The model under review builds one solid part; all positions refer to its coordinate system, in mm. Round coordinates to 2 decimals unless told otherwise and drop trailing zeros. Write each loop counter-clockwise with the first axis right and the second up, starting at its lowest first coordinate (ties: lowest second). Pieces come first, ordered by that corner, then holes. Notation, with made-up numbers: M 57.25,-9 L 92.25,-9 A20 cw 92.25,26 Z; hole C 70.25,-31 d6. An arc over 180 degrees is marked long. Write item = value, one per line. Start each with the question number.
Item 1: Take a section at B-B, the plane z = 4. Give the boundary of the cut face in (x, y), plus the area to 3 significant figures.
Item 2: Take a section at D-D, the plane y = 58.5. Give the boundary of the cut face in (x, z).
Item 3: To check wall thickness, follow line 1 along Z through (x, y) = (70.5, 58.5); line 2 along Z through (x, y) = (70.5, 59); line 3 along Y through (x, z) = (72, 4.5). State the ranges of each line that lie inside material, in increasing order.
Item 4: Take a section at C-C, the plane x = 71.25. Give the number of separate pieces and of enclosed holes in the cut face, plus the area to 3 significant figures.
Item 5: Take a section at A-A, the plane y = 52. Give the boundary of the cut face in (x, z).
Item 6: The part is to be moulded in two halves that separate along Z. For faces 1 (the cylindrical face through (70.04, 78.54, 4.95)), 2 (the flat face through (70, 65, 0)), 3 (the cylindrical face through (70.04, 67.16, 5.06)), say which applies: +Z half, -Z half, draft (parallel to the pull), parting line (faces both ways), or undercut.
Item 7: For pin 1 Ø1.5 at (x, z) = (71.5, 2) entering from +Y; pin 2 Ø1.4 at (x, y) = (71.08, 72.9) entering from +Z; pin 3 Ø3 at (x, z) = (70.5, 2) entering from +Y; pin 4 Ø1.5 at (y, z) = (75, 3) entering from +X, all flat-tipped, find the tip position at first contact; note any pin that passes through.
from build123d import *

# Parameters (mm, degrees)
SKETCH1_R           = 1.2065
BOSS_EXTRUDE1_DEPTH = 10.033
CUT_EXTRUDE1_DEPTH  = 10.033
CUT_EXTRUDE2_DEPTH  = 10.033


with BuildPart() as part:
    # Sketch1 → Boss-Extrude1 (new body)
    with BuildSketch(Plane.XY):
        with BuildLine():
            Line((74.127846298, 88.795942837), (72.00043944, 36.574422097))
            ThreePointArc((72.00043944, 36.574422097), (66.89810991, 60.973237803), (68.966334727, 85.813898433))
            ThreePointArc((68.966334727, 85.813898433), (71.21567331, 87.878558548), (74.127846298, 88.795942837))
        make_face()
        with Locations((70.925382829, 77.722422097)):
            Circle(SKETCH1_R, mode=Mode.SUBTRACT)
        with Locations((71.077782829, 72.896422097)):
            Circle(SKETCH1_R, mode=Mode.SUBTRACT)
    extrude(amount=BOSS_EXTRUDE1_DEPTH)

    # Sketch2 → Cut-Extrude1 (cut)
    with BuildSketch(Plane(origin=(70.393641123, -2.867704976, 0), x_dir=(0, 0, -1), z_dir=(0.999171234, -0.040704363, 0))):
        with BuildLine():
            Line((-1.27, 39.474842481), (-8.763, 39.474842481))
            Line((-8.763, 39.474842481), (-6.9215, 68.049842481))
            ThreePointArc((-6.9215, 68.049842481), (-5.0165, 69.954842481), (-3.1115, 68.049842481))
            Line((-3.1115, 68.049842481), (-1.27, 39.474842481))
        make_face()
    extrude(amount=-CUT_EXTRUDE1_DEPTH, mode=Mode.SUBTRACT)

    # Sketch3 → Cut-Extrude2 (cut)
    with BuildSketch(Plane.XY.offset(10.033)):
        with BuildLine():
            Line((70.704380761, 40.389805653), (72.155871014, 40.389805653))
            Line((72.155871014, 40.389805653), (72.00043944, 36.574422097))
            ThreePointArc((72.00043944, 36.574422097), (71.330186821, 38.474564785), (70.704380761, 40.389805653))
        make_face()
    extrude(amount=-CUT_EXTRUDE2_DEPTH, mode=Mode.SUBTRACT)


solid = part.part
Response values:
q1.outline = M 66.74,67 L 73.23,66.74 L 74.13,88.8 A7.04 ccw 68.97,85.81 A86.49 ccw Z; hole C 70.93,77.72 d2.41; hole C 71.08,72.9 d2.41
q1.area = 117 mm2
q2.outline = M 67.09,0 L 72.89,0 L 72.89,2.68 L 67.09,2.67 Z; M 67.09,7.36 L 72.89,7.35 L 72.89,10.03 L 67.09,10.03 Z
q3.line_1 = 0 to 2.68, 7.36 to 10.03
q3.line_2 = 0 to 2.71, 7.32 to 10.03
q3.line_3 = 67.01 to 72.12, 73.67 to 77.17, 78.27 to 88.27
q4.separate_pieces = 3
q4.enclosed_holes = 0
q4.area = 289 mm2
q5.outline = M 67.92,0 L 72.63,0 L 72.63,2.26 L 67.92,2.25 Z; M 67.92,7.78 L 72.63,7.77 L 72.63,10.03 L 67.92,10.03 Z
q6.face_1 = draft
q6.face_2 = -Z half
q6.face_3 = undercut
q7.pin_1 = 88.37
q7.pin_2 = through
q7.pin_3 = 88.27
q7.pin_4 = 73.6
